```python
from build123d import *

# Parameters (mm, degrees)
BOSS_EXTRUDE1_DEPTH  = 2
FILLET1_R            = 1
SKETCH2_W            = 1.5
SKETCH2_H            = 3.5
CUT_EXTRUDE1_DEPTH   = 44.710525048
BOSS_EXTRUDE2_START  = 2
BOSS_EXTRUDE2_DEPTH  = 2
SKETCH6_R            = 1.5
CUT_EXTRUDE2_DEPTH   = 14
FILLET1_OF_MIRROR1_R = 1


with BuildPart() as part:
    # Sketch1 → Boss-Extrude1 (new body)
    with BuildSketch(Plane(origin=(0, 0, 0), x_dir=(1, 0, 0), z_dir=(0, 1, 0))):
        Polygon((0, -4), (0, 4), (33.1, 4), (33.1, 7), (43.1, 7), (43.1, -7), (33.1, -7), (33.1, -4), align=None)
    boss_extrude1 = extrude(amount=BOSS_EXTRUDE1_DEPTH)

    # Fillet1
    fillet1_edges = [part.edges().sort_by_distance(p)[0] for p in [
        (33.1, 1, -4),
        (33.1, 1, -7),
        (43.1, 1, -7),
        (43.1, 1, 7),
        (33.1, 1, 7),
        (33.1, 1, 4),
    ]]
    fillet(fillet1_edges, radius=FILLET1_R)

    # Sketch2 → Cut-Extrude1 (cut, through all)
    with BuildSketch(Plane(origin=(0, 2, 0), x_dir=(1, 0, 0), z_dir=(0, 1, 0))):
        with Locations((35.85, -3.25)):
            Rectangle(SKETCH2_W, SKETCH2_H)
        with Locations((40.35, 3.25)):
            Rectangle(SKETCH2_W, SKETCH2_H)
        with Locations((40.35, -3.25)):
            Rectangle(SKETCH2_W, SKETCH2_H)
        with Locations((35.85, 3.25)):
            Rectangle(SKETCH2_W, SKETCH2_H)
    cut_extrude1 = extrude(amount=-CUT_EXTRUDE1_DEPTH, mode=Mode.SUBTRACT)

    # Sketch5 → Boss-Extrude2 (add)
    with BuildSketch(Plane(origin=(0, 2, 0), x_dir=(1, 0, 0), z_dir=(0, 1, 0)).offset(BOSS_EXTRUDE2_START)):
        with BuildLine():
            Line((0, -2), (32.1, -2))
            ThreePointArc((32.1, -2), (34.221320344, -2.878679656), (35.1, -5))
            Line((35.1, -5), (41.1, -5))
            Line((41.1, -5), (41.1, 5))
            Line((41.1, 5), (35.1, 5))
            ThreePointArc((35.1, 5), (34.221320344, 2.878679656), (32.1, 2))
            Line((32.1, 2), (0, 2))
            Line((0, 2), (0, 4))
            Line((0, 4), (32.1, 4))
            ThreePointArc((32.1, 4), (32.807106781, 4.292893219), (33.1, 5))
            Line((33.1, 5), (33.1, 6))
            ThreePointArc((33.1, 6), (33.392893219, 6.707106781), (34.1, 7))
            Line((34.1, 7), (42.1, 7))
            ThreePointArc((42.1, 7), (42.807106781, 6.707106781), (43.1, 6))
            Line((43.1, 6), (43.1, -6))
            ThreePointArc((43.1, -6), (42.807106781, -6.707106781), (42.1, -7))
            Line((42.1, -7), (34.1, -7))
            ThreePointArc((34.1, -7), (33.392893219, -6.707106781), (33.1, -6))
            Line((33.1, -6), (33.1, -5))
            ThreePointArc((33.1, -5), (32.807106781, -4.292893219), (32.1, -4))
            Line((32.1, -4), (0, -4))
            Line((0, -4), (0, -2))
        make_face()
    boss_extrude2 = extrude(amount=-BOSS_EXTRUDE2_DEPTH)

    # Sketch6 → Cut-Extrude2 (cut)
    with BuildSketch(Plane.XY.offset(7)):
        with Locations((38.1, 3.5)):
            Circle(SKETCH6_R)
    cut_extrude2 = extrude(amount=-CUT_EXTRUDE2_DEPTH, mode=Mode.SUBTRACT)

    # Mirror1: Boss-Extrude1, Cut-Extrude1, Boss-Extrude2, Cut-Extrude2 across plane
    add(boss_extrude1.mirror(Plane(origin=(0, 0, 0), x_dir=(0, 0, 1), z_dir=(1, 0, 0))))
    add(cut_extrude1.mirror(Plane(origin=(0, 0, 0), x_dir=(0, 0, 1), z_dir=(1, 0, 0))), mode=Mode.SUBTRACT)
    add(boss_extrude2.mirror(Plane(origin=(0, 0, 0), x_dir=(0, 0, 1), z_dir=(1, 0, 0))))
    add(cut_extrude2.mirror(Plane(origin=(0, 0, 0), x_dir=(0, 0, 1), z_dir=(1, 0, 0))), mode=Mode.SUBTRACT)

    # Fillet1 of Mirror1
    fillet1_of_mirror1_edges = [part.edges().sort_by_distance(p)[0] for p in [
        (-33.1, 1, -4),
        (-33.1, 1, -7),
        (-43.1, 1, -7),
        (-43.1, 1, 7),
        (-33.1, 1, 7),
        (-33.1, 1, 4),
    ]]
    fillet(fillet1_of_mirror1_edges, radius=FILLET1_OF_MIRROR1_R)


solid = part.part
```
The model under review builds one solid part; all positions refer to its coordinate system, in mm. A direction names the side the tool comes from. Round coordinates to 2 decimals unless told otherwise and drop trailing zeros. Loops run counter-clockwise (first coordinate to the right, second up) from the corner with the lowest first, then second, coordinate; pieces in that order, holes last. Notation, with made-up numbers: (17.5, 22) -> (28.5, 22) arc R31 ccw to (28.5, 60) -> close; hole circle Ø6 at (44, -27). An arc over 180 degrees is marked (long way). Answer as a JSON object with one key per item and string values. Group by question number.
1) For pin 1 Ø1.6 at (x, y) = (-7.5, 3) entering from +Z; pin 2 Ø1.5 at (x, y) = (-31, 0.5) entering from -Z, all flat-tipped, find the tip position at first contact; note any pin that passes through.
2) We need section A-A on x = 19.5. Write out the cut boundary in (y, z), then the cut area to 3 significant figures.
3) For line 1 (X direction, y = 3.5, z = -5.35); line 2 (X direction, y = 2.25, z = -2.75); line 3 (X direction, y = 1.1, z = -2.75), list the stretches that pass through material, from the lowest coordinate up. Write a range as [from, to].
4) Mouldability with a two-part tool opening along X and no side actions: class faces 1 (the face through (-40, 2, -5)), 2 (the face through (-38.2, 1.6, 7)), 3 (the face through (-43.1, 2, 0)) as released by +X, released by -X, zero draft, split by the parting line, or undercut.
5) For faces 4 (the face through (36.6, 1, 3)), 5 (the face through (-1, 0, 0)), 6 (the face through (0, 3, -2)), list the 3-axis set-ups (+Z, -Z, +X, -X, +Y, -Y) from which the entire face can be reached by the end or side of a thin tool; tool diameter is ignored.
Result set:
{
 "1": {"pin 1": "z = 4", "pin 2": "z = -4"},
 "2": {"outline": "(0, -4) -> (4, -4) -> (4, -2) -> (2, -2) -> (2, 2) -> (4, 2) -> (4, 4) -> (0, 4) -> close", "area": "24.0 mm²"},
 "3": {"line 1": "[-43.1, -39.6], [-36.6, -33.1], [33.1, 36.6], [39.6, 43.1]", "line 2": "[-43.1, -41.1], [-34.08, 34.08], [41.1, 43.1]", "line 3": "[-43.1, -41.1], [-39.6, -36.6], [-35.1, 35.1], [36.6, 39.6], [41.1, 43.1]"},
 "4": {"face 1": "undercut", "face 2": "zero draft", "face 3": "released by -X"},
 "5": {"face 4": "+Y, -Y", "face 5": "+Z, -Z, +X, -X, -Y", "face 6": "+Y"}
}
